Build history of the part. All positions in model axes, mm. A direction names the side the tool comes from. Round coordinates to 2 decimals unless told otherwise and drop trailing zeros. Write each loop counter-clockwise with the first axis right and the second up, starting at its lowest first coordinate (ties: lowest second). Pieces come first, ordered by that corner, then holes.
1) Which spindle directions (+Z, -Z, +X, -X, +Y, -Y) get a long thin tool onto all of the face, cutting with end or side? Do faces 1 (the flat face through (132.884, 23.436, -230.162)), 2 (the flat face through (-2, 12, -240.487)). Say none if no direction does.
2) Saw through at B-B (x = -59.5). Write the cut outline in (y, z).
3) Saw through at A-A (y = 11.5). Write the cut outline in (x, z), plus the area to 3 significant figures.
4) Wall check: probe 1 along Z at (x, y) = (84, 7.25); probe 2 along Y at (x, z) = (-52.5, -236.25); probe 3 along X at (y, z) = (1, -219.5). Give the ranges that are in metal, low to high.
5) Pull direction Y, two halves, no side cores. Call faces 3 (the flat face through (2, 12, -219.487)), 4 (the flat face through (2, 25, -230)), 5 (the flat face through (-132.68, 23.44, -229.81)): +Y half, -Y half, draft (parallel to the pull), parting line (faces both ways), or undercut.
6) Saw through at C-C (z = -238). Write the cut outline in (x, y), plus the area to 3 significant figures.
from build123d import *

# Parameters (mm, degrees)
BOSS_EXTRUDE1_DEPTH = 25
SHELL1_T            = -2
SKETCH2_R           = 5
CUT_EXTRUDE1_DEPTH  = 53


with BuildPart() as part:
    # Sketch1 → Boss-Extrude1 (new body)
    with BuildSketch(Plane(origin=(0, 0, 0), x_dir=(1, 0, 0), z_dir=(0, 1, 0))):
        Polygon((125.56624327, 217.48711306), (-125.56624327, 217.48711306), (-140, 242.48711306), (140, 242.48711306), align=None)
    extrude(amount=BOSS_EXTRUDE1_DEPTH)

    # Shell1
    shell1_openings = [part.faces().sort_by_distance(p)[0] for p in [
        (-132.783121635, 12.5, -229.98711306),
        (132.783121635, 12.5, -229.98711306),
    ]]
    offset(amount=SHELL1_T, openings=shell1_openings, kind=Kind.INTERSECTION)

    # Sketch2 → Cut-Extrude1 (cut)
    with BuildSketch(Plane(origin=(0, 25, 0), x_dir=(1, 0, 0), z_dir=(0, 1, 0))):
        with Locations((47.783121635, 228.657359562)):
            Circle(SKETCH2_R)
    extrude(amount=-CUT_EXTRUDE1_DEPTH, mode=Mode.SUBTRACT)


solid = part.part
Evaluation:
1. face 1: +Z, +X, +Y, -Y
1. face 2: +X, -X
2. outline: (0, -242.49) - (25, -242.49) - (25, -217.49) - (0, -217.49) - close; hole (2, -240.49) - (23, -240.49) - (23, -219.49) - (2, -219.49) - close
3. outline: (-140, -242.49) - (140, -242.49) - (138.85, -240.49) - (-138.85, -240.49) - close; (-126.72, -219.49) - (126.72, -219.49) - (125.57, -217.49) - (-125.57, -217.49) - close
3. area: 1,060 mm2
4. probe 1: z = -242.49 to -240.49, -219.49 to -217.49
4. probe 2: y = 0 to 2, 23 to 25
4. probe 3: x = -126.73 to 126.73
5. face 3: undercut
5. face 4: +Y half
5. face 5: draft
6. outline: (-137.41, 0) - (137.41, 0) - (137.41, 2) - (-137.41, 2) - close; (-137.41, 23) - (137.41, 23) - (137.41, 25) - (-137.41, 25) - close
6. area: 1,100 mm2
